The listing builds one solid part. Answer for the finished solid, in the listing's coordinates (mm). Face numbers are marked on the shaded views. A direction names the side the tool comes from. Give positions to 0.01 mm unless a question says otherwise; leave off trailing zeros. Write each loop counter-clockwise with the first axis right and the second up, starting at its lowest first coordinate (ties: lowest second). Pieces come first, ordered by that corner, then holes. Notation, with made-up numbers: M 23.25,22.25 L 49.25,22.25 A24 ccw 49.25,57.25 Z; hole C 53.25,38.25 d10. An arc over 180 degrees is marked long. Answer as a JSON object with one key per item and string values.
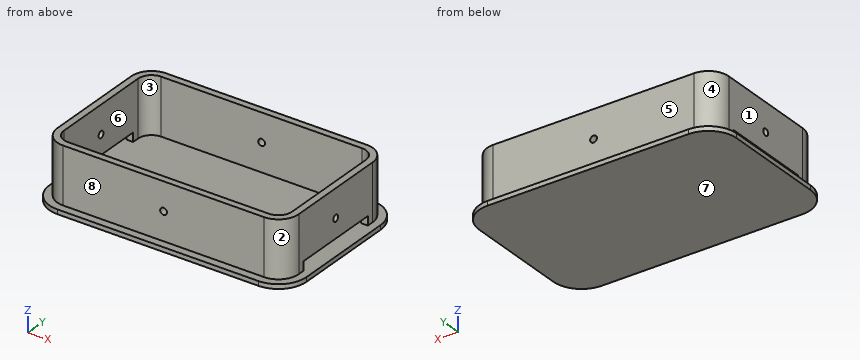
```python
from build123d import *

# Parameters (mm, degrees)
PAD001_DEPTH         = 2
PAD003_DEPTH         = 27
SKETCH_R             = 1.5
POCKET_DEPTH         = 309.479101
SKETCH004_W          = 40
SKETCH004_H          = 4
POCKET001_DEPTH      = 57.001
POCKET001_DEPTH_BACK = -57.001
POLARPATTERN_COUNT   = 4


with BuildPart() as part:
    # Sketch001 → Pad001 (new body)
    with BuildSketch(Plane.XY):
        with BuildLine():
            Line((-57, 23), (-57, -23))
            ThreePointArc((-57, -23), (-53.338835, -31.838835), (-44.5, -35.5))
            Line((-44.5, -35.5), (44.5, -35.5))
            ThreePointArc((44.5, -35.5), (53.338835, -31.838835), (57, -23))
            Line((57, -23), (57, 23))
            ThreePointArc((57, 23), (53.338835, 31.838835), (44.5, 35.5))
            Line((44.5, 35.5), (-44.5, 35.5))
            ThreePointArc((-44.5, 35.5), (-53.338835, 31.838835), (-57, 23))
        make_face()
    extrude(amount=PAD001_DEPTH)

    # Sketch003 → Pad003 (join)
    with BuildSketch(Plane.XY):
        with BuildLine():
            Line((-44.5, 32), (44.5, 32))
            ThreePointArc((53.5, 23), (50.863961, 29.363961), (44.5, 32))
            Line((53.5, 23), (53.5, -23))
            ThreePointArc((44.5, -32), (50.863961, -29.363961), (53.5, -23))
            Line((44.5, -32), (-44.5, -32))
            ThreePointArc((-53.5, -23), (-50.863961, -29.363961), (-44.5, -32))
            Line((-53.5, -23), (-53.5, 23))
            ThreePointArc((-44.5, 32), (-50.863961, 29.363961), (-53.5, 23))
        make_face()
        with BuildLine():
            Line((-50.5, 23), (-50.5, -23))
            ThreePointArc((-50.5, -23), (-48.742641, -27.242641), (-44.5, -29))
            Line((-44.5, -29), (44.5, -29))
            ThreePointArc((44.5, -29), (48.742641, -27.242641), (50.5, -23))
            Line((50.5, -23), (50.5, 23))
            ThreePointArc((50.5, 23), (48.742641, 27.242641), (44.5, 29))
            Line((44.5, 29), (-44.5, 29))
            ThreePointArc((-44.5, 29), (-48.742641, 27.242641), (-50.5, 23))
        make_face(mode=Mode.SUBTRACT)
    extrude(amount=PAD003_DEPTH)

    # Sketch → Pocket (cut, through all)
    with BuildSketch(Plane.XZ):
        with Locations((0, 14.5)):
            Circle(SKETCH_R)
    pocket = extrude(amount=-POCKET_DEPTH, mode=Mode.SUBTRACT)

    # Sketch004 → Pocket001 (cut, two sides)
    with BuildSketch(Plane.YZ) as pocket001_sk:
        with Locations((0, 4)):
            Rectangle(SKETCH004_W, SKETCH004_H)
    extrude(amount=-POCKET001_DEPTH, mode=Mode.SUBTRACT)
    extrude(pocket001_sk.sketch, amount=-POCKET001_DEPTH_BACK, mode=Mode.SUBTRACT)

    # PolarPattern: Pocket ×4 about axis
    polarpattern_axis = Axis((0, 0, 0), (0, 0, 1))
    for i in range(1, POLARPATTERN_COUNT):
        add(pocket.rotate(polarpattern_axis, i * 360 / POLARPATTERN_COUNT), mode=Mode.SUBTRACT)


solid = part.part
```
1. The mould has two halves that part along Y. Classify the marked faces 6, 7 and 8: released by +Y, released by -Y, zero draft, split by the parting line, or undercut.
Verdict:
{"face 6": "undercut", "face 7": "zero draft", "face 8": "released by -Y"}
2. A cutting plane is placed at D-D, the plane y = 18.5. Give the vertices of the cut face in (x, z), plus the area to 3 significant figures.
Verdict:
{"outline": "M -57,0 L 57,0 L 57,2 L -57,2 Z; M -53.5,6 L -50.5,6 L -50.5,27 L -53.5,27 Z; M 50.5,6 L 53.5,6 L 53.5,27 L 50.5,27 Z", "area": "354 mm2"}
3. Flat-ended cylindrical pins translate along their axes: pin 1 (2.5 mm diameter, centred on x = 51.5, y = -3, fed in from -Z); pin 2 (6 mm diameter, centred on x = -30.5, y = 10, fed in from +Z); pin 3 (1.5 mm diameter, centred on x = -52.5, z = 4, fed in from +Y); pin 4 (12.5 mm diameter, centred on x = 16, z = 12.5, fed in from +Y). Find the tip coordinate at first contact, or state that the pin passes through.
Verdict:
{"pin 1": "stops at z = 0", "pin 2": "stops at z = 2", "pin 3": "stops at y = 28.33", "pin 4": "stops at y = 32"}
4. Consider line 1 along Z through (x, y) = (51.6, 0); line 2 along Y through (x, z) = (3.5, 21.75); line 3 along X through (y, z) = (-5.5, 13.25). Determine where each line is inside the solid, lowest interval first.
Verdict:
{"line 1": "z = 0 to 2, 6 to 13, 16 to 27", "line 2": "y = -32 to -29, 29 to 32", "line 3": "x = -53.5 to -50.5, 50.5 to 53.5"}
5. A cutting plane is placed at A-A, the plane y = 0. Give the vertices of the cut face in (x, z).
Verdict:
{"outline": "M -57,0 L 57,0 L 57,2 L -57,2 Z; M -53.5,6 L -50.5,6 L -50.5,13 L -53.5,13 Z; M -53.5,16 L -50.5,16 L -50.5,27 L -53.5,27 Z; M 50.5,6 L 53.5,6 L 53.5,13 L 50.5,13 Z; M 50.5,16 L 53.5,16 L 53.5,27 L 50.5,27 Z"}
6. A cutting plane is placed at C-C, the plane z = 8.5. Give the vertices of the cut face in (x, y), plus the area to 3 significant figures.
Verdict:
{"outline": "M -53.5,-23 A9 ccw -44.5,-32 L 44.5,-32 A9 ccw 53.5,-23 L 53.5,23 A9 ccw 44.5,32 L -44.5,32 A9 ccw -53.5,23 Z; hole M -50.5,-23 A6 ccw -44.5,-29 L 44.5,-29 A6 ccw 50.5,-23 L 50.5,23 A6 ccw 44.5,29 L -44.5,29 A6 ccw -50.5,23 Z", "area": "951 mm2"}
7. For the marked faces 1, 2, 3, 4 and 5, determine the directions among +Z, -Z, +X, -X, +Y, -Y from which every point of the face is accessible in a straight line to the end or side of a thin tool.
Verdict:
{"face 1": "+Z, -X, +Y, -Y", "face 2": "+Z, +X, -Y", "face 3": "+Z", "face 4": "+Z, -X, +Y", "face 5": "+Z, +X, -X, +Y"}
8. A cutting plane is placed at B-B, the plane x = 0. Give the vertices of the cut face in (y, z).
Verdict:
{"outline": "M -35.5,0 L 35.5,0 L 35.5,2 L 32,2 L 32,13 L 29,13 L 29,2 L -29,2 L -29,13 L -32,13 L -32,2 L -35.5,2 Z; M -32,16 L -29,16 L -29,27 L -32,27 Z; M 29,16 L 32,16 L 32,27 L 29,27 Z"}
